Autodesk Fusion 360 part; units mm, degrees
sketch "Sketch1" plane through (0, 0, 0) normal (0, 0, 1) x (1, 0, 0)
  line L0 (2, 0) -> (126.53, 0)
  line L1 (128.53, 2) -> (128.53, 128)
  line L2 (126.53, 130) -> (2, 130)
  line L3 (0, 128) -> (0, 2)
  line L4 (0, 70) -> (128.53, 70) construction
  line L5 (0, 46.94) -> (128.53, 46.94) construction
  line L6 (0, 92) -> (128.53, 92) construction
  line L7 (0, 20) -> (128.53, 20) construction
  line L8 (2.5, 130) -> (2.5, 0) construction
  line L9 (126.03, 130) -> (126.03, 0) construction
  circle A0 centre (71, 46.94) radius 3.55
  circle A1 centre (17, 46.94) radius 3.55
  circle A2 centre (84.5, 46.94) radius 3.55
  circle A3 centre (30.5, 46.94) radius 3.55
  circle A4 centre (111.53, 46.94) radius 3.55
  circle A5 centre (44, 46.94) radius 3.55
  circle A6 centre (57.5, 46.94) radius 3.55
  circle A7 centre (126.03, 92) radius 1.5
  circle A8 centre (2.5, 92) radius 1.5
  circle A9 centre (2.5, 20) radius 1.5
  circle A10 centre (126.03, 20) radius 1.5
  line L10 (107.73, 62.5) -> (101.33, 62.5)
  line L11 (99.03, 64.8) -> (99.03, 75.2)
  line L12 (101.33, 77.5) -> (107.73, 77.5)
  line L13 (110.03, 75.2) -> (110.03, 64.8)
  line L14 (110.03, 62.5) -> (99.03, 77.5) construction
  line L15 (99.03, 62.5) -> (110.03, 77.5) construction
  line L16 (88.03, 62.5) -> (81.33, 62.5)
  line L17 (79.03, 64.8) -> (79.03, 75.5)
  line L18 (81.03, 77.5) -> (88.03, 77.5)
  line L19 (90.03, 75.5) -> (90.03, 64.5)
  line L20 (90.03, 62.5) -> (79.03, 77.5) construction
  line L21 (79.03, 62.5) -> (90.03, 77.5) construction
  line L22 (70.03, 61.5) -> (59.03, 61.5)
  line L23 (57.03, 63.5) -> (57.03, 76.5)
  line L24 (59.03, 78.5) -> (70.03, 78.5)
  line L25 (72.03, 76.5) -> (72.03, 63.5)
  line L26 (72.03, 61.5) -> (57.03, 78.5) construction
  line L27 (57.03, 61.5) -> (72.03, 78.5) construction
  line L28 (46.53, 62) -> (18.53, 62)
  line L29 (16.53, 64) -> (16.53, 76)
  line L30 (18.53, 78) -> (46.53, 78)
  line L31 (48.53, 76) -> (48.53, 64)
  line L32 (48.53, 62) -> (16.53, 78) construction
  line L33 (16.53, 62) -> (48.53, 78) construction
  line L34 (100.23, 49.94) -> (94.83, 49.94)
  line L35 (92.53, 47.64) -> (92.53, 46.24)
  line L36 (94.83, 43.94) -> (100.23, 43.94)
  line L37 (102.53, 46.24) -> (102.53, 47.64)
  line L38 (102.53, 49.94) -> (92.53, 43.94) construction
  line L39 (92.53, 49.94) -> (102.53, 43.94) construction
  arc A11 (2, 130) -> (0, 128) centre (2, 128) ccw
  arc A12 (128.53, 128) -> (126.53, 130) centre (126.53, 128) ccw
  arc A13 (126.53, 0) -> (128.53, 2) centre (126.53, 2) ccw
  arc A14 (0, 2) -> (2, 0) centre (2, 2) ccw
  arc A15 (18.53, 78) -> (16.53, 76) centre (18.53, 76) ccw
  arc A16 (46.53, 62) -> (48.53, 64) centre (46.53, 64) ccw
  arc A17 (16.53, 64) -> (18.53, 62) centre (18.53, 64) ccw
  arc A18 (48.53, 76) -> (46.53, 78) centre (46.53, 76) ccw
  arc A19 (59.03, 78.5) -> (57.03, 76.5) centre (59.03, 76.5) ccw
  arc A20 (72.03, 76.5) -> (70.03, 78.5) centre (70.03, 76.5) ccw
  arc A21 (70.03, 61.5) -> (72.03, 63.5) centre (70.03, 63.5) ccw
  arc A22 (57.03, 63.5) -> (59.03, 61.5) centre (59.03, 63.5) ccw
  arc A23 (81.03, 77.5) -> (79.03, 75.5) centre (81.03, 75.5) ccw
  arc A24 (90.03, 75.5) -> (88.03, 77.5) centre (88.03, 75.5) ccw
  arc A25 (88.03, 62.5) -> (90.03, 64.5) centre (88.03, 64.5) ccw
  arc A26 (79.03, 64.8) -> (81.33, 62.5) centre (81.33, 64.8) ccw
  arc A27 (101.33, 77.5) -> (99.03, 75.2) centre (101.33, 75.2) ccw
  arc A28 (110.03, 75.2) -> (107.73, 77.5) centre (107.73, 75.2) ccw
  arc A29 (107.73, 62.5) -> (110.03, 64.8) centre (107.73, 64.8) ccw
  arc A30 (99.03, 64.8) -> (101.33, 62.5) centre (101.33, 64.8) ccw
  arc A31 (94.83, 49.94) -> (92.53, 47.64) centre (94.83, 47.64) ccw
  arc A32 (102.53, 47.64) -> (100.23, 49.94) centre (100.23, 47.64) ccw
  arc A33 (92.53, 46.24) -> (94.83, 43.94) centre (94.83, 46.24) ccw
  arc A34 (100.23, 43.94) -> (102.53, 46.24) centre (100.23, 46.24) ccw
  line L40 (0, 126.5) -> (128.53, 126.5) construction
  line L41 (0, 3.5) -> (128.53, 3.5) construction
  line L42 (118.53, 130) -> (118.53, 0) construction
  line L43 (10, 130) -> (10, 0) construction
  circle A35 centre (10, 126.5) radius 2
  circle A36 centre (118.53, 126.5) radius 2
  circle A37 centre (10, 3.5) radius 2
  circle A38 centre (118.53, 3.5) radius 2
  line L44 (0, 28) -> (128.53, 28) construction
  line L45 (109.765, 20.75) -> (18.765, 20.75)
  line L46 (16.765, 22.75) -> (16.765, 33.25)
  line L47 (18.765, 35.25) -> (109.765, 35.25)
  line L48 (111.765, 33.25) -> (111.765, 22.75)
  line L49 (111.765, 20.75) -> (16.765, 35.25) construction
  line L50 (16.765, 20.75) -> (111.765, 35.25) construction
  arc A39 (18.765, 35.25) -> (16.765, 33.25) centre (18.765, 33.25) ccw
  arc A40 (111.765, 33.25) -> (109.765, 35.25) centre (109.765, 33.25) ccw
  arc A41 (16.765, 22.75) -> (18.765, 20.75) centre (18.765, 22.75) ccw
  arc A42 (109.765, 20.75) -> (111.765, 22.75) centre (109.765, 22.75) ccw
  line L51 (0, 113.5) -> (128.53, 113.5) construction
  line L52 (0, 102) -> (128.53, 102) construction
  circle A43 centre (106.03, 113.5) radius 3.25
  circle A44 centre (106.03, 102) radius 3.25
  circle A45 centre (71.03, 113.5) radius 3.25
  circle A46 centre (71.03, 102) radius 3.25
  circle A47 centre (36.03, 113.5) radius 3.25
  line L53 (0, 51.84) -> (128.53, 51.84) construction
  circle A48 centre (17, 51.84) radius 0.75
  circle A49 centre (30.5, 51.84) radius 0.75
  circle A50 centre (44, 51.84) radius 0.75
  circle A51 centre (57.5, 51.84) radius 0.75
  circle A52 centre (71, 51.84) radius 0.75
  circle A53 centre (84.5, 51.84) radius 0.75
  circle A54 centre (111.53, 51.84) radius 0.75
  point P0 (128.53, 0)
  point P1 (0, 130)
  point P2 (104.53, 70)
  point P3 (84.53, 70)
  point P4 (64.53, 70)
  point P5 (32.53, 70)
  point P6 (97.53, 46.94)
  point P7 (64.265, 28)
  dimension "d1" = 128.53
  dimension "d2" = 130
  dimension "d4" = 2.5
  dimension "d5" = 2.5
  dimension "d7" = 60
  dimension "d25" = 7.1
  dimension "d26" = 7.1
  dimension "d27" = 7.1
  dimension "d28" = 7.1
  dimension "d29" = 7.1
  dimension "d30" = 7.1
  dimension "d31" = 7.1
  dimension "d32" = 17
  dimension "d33" = 13.5
  dimension "d34" = 13.5
  dimension "d35" = 13.5
  dimension "d36" = 13.5
  dimension "d37" = 13.5
  dimension "d38" = 17
  dimension "d42" = 3
  dimension "d43" = 3
  dimension "d44" = 3
  dimension "d45" = 3
  dimension "d49" = 72
  dimension "d54" = 23.06
  dimension "d55" = 22
  dimension "d56" = 11
  dimension "d57" = 15
  dimension "d58" = 24
  dimension "d59" = 11
  dimension "d60" = 15
  dimension "d61" = 20
  dimension "d62" = 15
  dimension "d63" = 17
  dimension "d64" = 20
  dimension "d65" = 32
  dimension "d66" = 16
  dimension "d67" = 32
  dimension "d68" = 10
  dimension "d69" = 6
  dimension "d70" = 14
  dimension "d75" = 2
  dimension "d76" = 2
  dimension "d77" = 2
  dimension "d78" = 2
  dimension "d79" = 2
  dimension "d80" = 2
  dimension "d81" = 2
  dimension "d82" = 2
  dimension "d83" = 2
  dimension "d84" = 2
  dimension "d85" = 2.3
  dimension "d86" = 123
  dimension "d87" = 3.5
  dimension "d89" = 4
  dimension "d90" = 4
  dimension "d91" = 4
  dimension "d92" = 4
  dimension "d93" = 10
  dimension "d94" = 10
  dimension "d99" = 42
  dimension "d100" = 95
  dimension "d101" = 14.5
  dimension "d102" = 2
  dimension "d103" = 2
  dimension "d104" = 2
  dimension "d105" = 2
  dimension "d106" = 32
  dimension "d107" = 11.5
  dimension "d110" = 6.5
  dimension "d111" = 6.5
  dimension "d112" = 6.5
  dimension "d113" = 6.5
  dimension "d117" = 35
  dimension "d118" = 20
  dimension "d121" = 6.5
  dimension "d122" = 35
  dimension "d123" = 4.9
  dimension "d126" = 1.5
  dimension "d127" = 17
  dimension "d128" = 1.5
  dimension "d129" = 1.5
  dimension "d130" = 1.5
  dimension "d131" = 1.5
  dimension "d132" = 1.5
  dimension "d133" = 1.5
  dimension "d134" = 17
  dimension "d135" = 13.5
  dimension "d136" = 13.5
  dimension "d137" = 13.5
  dimension "d138" = 13.5
  dimension "d139" = 13.5
extrude "Extrude5" add sketch "Sketch1" along normal blind 1.5
equation "d7 = Offset_from_top"
equation "d25 = button_size"
equation "d26 = button_size"
equation "d27 = button_size"
equation "d28 = button_size"
equation "d29 = button_size"
equation "d30 = button_size"
equation "d31 = button_size"
equation "d33 = button_spacing"
equation "d34 = button_spacing"
equation "d35 = button_spacing"
equation "d36 = button_spacing"
equation "d37 = button_spacing"
equation "d42 = mount_hole"
equation "d43 = mount_hole"
equation "d44 = mount_hole"
equation "d45 = mount_hole"
equation "button_spacing = 13.5 mm"
equation "button_size = 7.1 mm"
equation "euro_screw_hole = 4 mm"
equation "d89 = euro_screw_hole"
equation "d90 = euro_screw_hole"
equation "d91 = euro_screw_hole"
equation "d92 = euro_screw_hole"
equation "mount_hole = 3 mm"
equation "Offset_from_top = 60 mm"
equation "audio_jack_hole = 6.5 mm"
equation "d110 = audio_jack_hole"
equation "d111 = audio_jack_hole"
equation "d112 = audio_jack_hole"
equation "d113 = audio_jack_hole"
equation "d121 = audio_jack_hole"
equation "led = 1.5 mm"
equation "d126 = led"
equation "d128 = led"
equation "d129 = led"
equation "d130 = led"
equation "d131 = led"
equation "d132 = led"
equation "d133 = led"
equation "d135 = button_spacing"
equation "d136 = button_spacing"
equation "d137 = button_spacing"
equation "d138 = button_spacing"
equation "d139 = button_spacing"
For this review, take the finished solid that the model builds, in its own axes (mm). Round coordinates to 2 decimals unless told otherwise and drop trailing zeros. Loops run counter-clockwise (first coordinate to the right, second up) from the corner with the lowest first, then second, coordinate; pieces in that order, holes last. Notation, with made-up numbers: (50.5, -34) - (105.5, -34) arc R31 cw to (105.5, -6) - close; hole circle Ø10 at (-21, 48). An arc over 180 degrees is marked (long way). One line per question, with ' | ' between items.
Q1. Take a section at B-B (y = 3.5). Give the boundary of the cut face in (x, z).
Taken from the geometry:
outline: (0, 0) - (8, 0) - (8, 1.5) - (0, 1.5) - close; (12, 0) - (116.53, 0) - (116.53, 1.5) - (12, 1.5) - close; (120.53, 0) - (128.53, 0) - (128.53, 1.5) - (120.53, 1.5) - close
Q2. Take a section at D-D (z = 0.3). State how many separate pieces and enclosed holes the cut face has, and give its area (3 significant figures).
Taken from the geometry:
separate pieces: 1 | enclosed holes: 33 | area: 13,700 mm²
Q3. Take a section at A-A (y = 28). Give the boundary of the cut face in (x, z) (3 decimals), and give its area (3 significant figures).
Taken from the geometry:
outline: (0, 0) - (16.765, 0) - (16.765, 1.5) - (0, 1.5) - close; (111.765, 0) - (128.53, 0) - (128.53, 1.5) - (111.765, 1.5) - close | area: 50.3 mm²
Q4. Take a section at C-C (x = 10). Give the boundary of the cut face in (y, z), and give its area (3 significant figures).
Taken from the geometry:
outline: (0, 0) - (1.5, 0) - (1.5, 1.5) - (0, 1.5) - close; (5.5, 0) - (124.5, 0) - (124.5, 1.5) - (5.5, 1.5) - close; (128.5, 0) - (130, 0) - (130, 1.5) - (128.5, 1.5) - close | area: 183 mm²
Q5. For line 1 along X through (y, z) = (71.5, 0.55); line 2 along Y through (x, z) = (30.5, 0.55); line 3 along Y through (x, z) = (10, 0.3), list the stretches that pass through material, from the lowest coordinate up. Write a range as [from, to].
Taken from the geometry:
line 1: x = [0, 16.53], [48.53, 57.03], [72.03, 79.03], [90.03, 99.03], [110.03, 128.53] | line 2: y = [0, 20.75], [35.25, 43.39], [50.49, 51.09], [52.59, 62], [78, 130] | line 3: y = [0, 1.5], [5.5, 124.5], [128.5, 130]
Q6. For pin 1 (2 mm diameter, centred on x = 88.5, y = 50, fed in from -Z), flat-tipped, find the tip position at first contact; note if it passes through.
Taken from the geometry:
pin 1: stops at z = 0
Q7. The part is to be moulded in two halves that separate along Y. For faces 1 (the cylindrical face through (87.78, 48.3, 0.74)), 2 (the flat face through (63, 80, 1.5)), say which applies: released by +Y, released by -Y, zero draft, split by the parting line, or undercut.
Taken from the geometry:
face 1: undercut | face 2: zero draft
